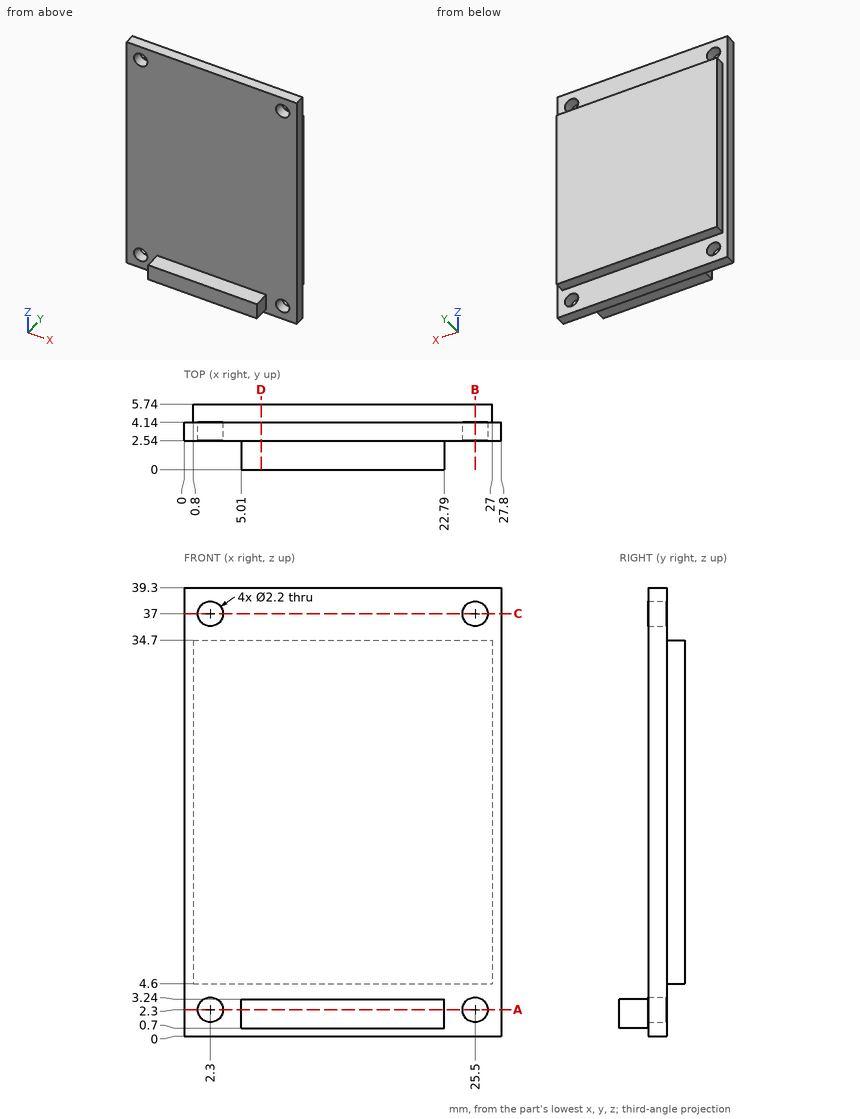
Geometry: see drawing. Coordinates: mm, zero at the bounding-box minimum. Round coordinates to 2 decimals unless told otherwise and drop trailing zeros. Loops run counter-clockwise (first coordinate to the right, second up) from the corner with the lowest first, then second, coordinate; pieces in that order, holes last. Notation, with made-up numbers: M 68.25,73 L 111.25,73 A20 cw 111.25,84 Z; hole C 24.25,75.25 d8. An arc over 180 degrees is marked long. Use a Markdown table: item, result. Add a question column.
1. Section query C-C on z = 37. Return the cut outline in (x, y), then the cut area to 3 significant figures.
2. Section query B-B on x = 25.5. Return the cut outline in (y, z), then the cut area to 3 significant figures.
3. Contact query for flat-ended pins moving along their axis: P1, Ø1.3, axis at y = 1, z = 2.5, coming from the +X side; P2, Ø2.5, axis at x = 25.5, z = 37, coming from the -Y side; P3, Ø1.3, axis at x = 10, y = 5, coming from the +Z side. Output: stop coordinate, or through.
4. Line query: line 1 (Z direction, x = 25.5, y = 3.1); line 2 (X direction, y = 3.2, z = 2.3); line 3 (Z direction, x = 26.25, y = 2.65). Output: solid intervals per line, ascending.
5. Section query D-D on x = 6.75. Return the cut outline in (y, z).
6. Section query A-A on z = 2.3. Return the cut outline in (x, y).
Reported:
| question | item | result |
|---|---|---|
| 1 | outline | M 0,2.54 L 1.2,2.54 L 1.2,4.14 L 0,4.14 Z; M 3.4,2.54 L 24.4,2.54 L 24.4,4.14 L 3.4,4.14 Z; M 26.6,2.54 L 27.8,2.54 L 27.8,4.14 L 26.6,4.14 Z |
| 1 | area | 37.4 mm² |
| 2 | outline | M 2.54,0 L 4.14,0 L 4.14,1.2 L 2.54,1.2 Z; M 2.54,3.4 L 4.14,3.4 L 4.14,4.6 L 5.74,4.6 L 5.74,34.7 L 4.14,34.7 L 4.14,35.9 L 2.54,35.9 Z; M 2.54,38.1 L 4.14,38.1 L 4.14,39.3 L 2.54,39.3 Z |
| 2 | area | 104 mm² |
| 3 | P1 | stops at x = 22.79 |
| 3 | P2 | stops at y = 2.54 |
| 3 | P3 | stops at z = 34.7 |
| 4 | line 1 | z = 0 to 1.2, 3.4 to 35.9, 38.1 to 39.3 |
| 4 | line 2 | x = 0 to 1.2, 3.4 to 24.4, 26.6 to 27.8 |
| 4 | line 3 | z = 0 to 1.5, 3.1 to 36.2, 37.8 to 39.3 |
| 5 | outline | M 0,0.7 L 2.54,0.7 L 2.54,0 L 4.14,0 L 4.14,4.6 L 5.74,4.6 L 5.74,34.7 L 4.14,34.7 L 4.14,39.3 L 2.54,39.3 L 2.54,3.24 L 0,3.24 Z |
| 6 | outline | M 0,2.54 L 1.2,2.54 L 1.2,4.14 L 0,4.14 Z; M 3.4,2.54 L 5.01,2.54 L 5.01,0 L 22.79,0 L 22.79,2.54 L 24.4,2.54 L 24.4,4.14 L 3.4,4.14 Z; M 26.6,2.54 L 27.8,2.54 L 27.8,4.14 L 26.6,4.14 Z |
